Geometry: final body of the model. Coordinates: model frame, mm. A direction names the side the tool comes from. Round coordinates to 2 decimals unless told otherwise and drop trailing zeros. Loops run counter-clockwise (first coordinate to the right, second up) from the corner with the lowest first, then second, coordinate; pieces in that order, holes last. Notation, with made-up numbers: (-2.75, 81.25) -> (33.25, 81.25) arc R8 ccw to (33.25, 86.25) -> close; hole circle Ø6 at (-19, 31). An arc over 180 degrees is marked (long way). Answer in a Markdown table with one row per item.
Autodesk Inventor part; units mm, degrees
ref_plane "Work Plane1" through (1.525, 0, 0) normal (0, 0, 1) x (1, 0, 0)
ref_plane "YZ Plane" through (0, 0, 0) normal (1, 0, 0) x (0, 1, 0)
ref_plane "XZ Plane" through (0, 0, 0) normal (0, 1, 0) x (-1, 0, 0)
sketch "Sketch1" plane through (0, 0, 0) normal (0, 0, 1) x (1, 0, 0)
  line L0 (0, 5.815) -> (0, 4)
  line L1 (38, 4) -> (60, 4)
  line L2 (60, 4) -> (60, 0)
  line L3 (60, 0) -> (-0.6001, 0)
  line L4 (-12.7201, 0) -> (72.12, 0)
  line L5 (-0.6001, 0) -> (-0.6001, 5.815)
  line L6 (-0.6001, 5.815) -> (0, 5.815)
  line L7 (38, 4) -> (37.2331, 4)
  line L8 (37.2331, 4) -> (0, 4)
  line L9 (0, -1.163) -> (0, 6.978)
  dimension "d0" = 60
  dimension "d1" = 22
  dimension "d2" = 8
  dimension "d9" = 0.6001
  dimension "d10" = 11.63
  dimension "d13" = 0.7669
  dimension "d14" = 8
revolve "Body" add sketch "Sketch1" angle 360 about axis through (60, 0, 0) along (-1, 0, 0)
sketch "Sketch2" plane through (-0.6001, 0, 0) normal (-1, 0, 0) x (0, 0, 1)
  line L0 (0, 7.5056) -> (6.5, 3.7528)
  line L1 (6.5, 3.7528) -> (6.5, -3.7528)
  line L2 (6.5, -3.7528) -> (0, -7.5056)
  line L3 (0, -7.5056) -> (-6.5, -3.7528)
  line L4 (-6.5, -3.7528) -> (-6.5, 3.7528)
  line L5 (-6.5, 3.7528) -> (0, 7.5056)
  point P0 (0, 0)
  point P1 (0, 0)
  dimension "d11" = 13
extrude "Head" add sketch "Sketch2" along normal blind 4.7
sketch "Sketch4" plane through (0, 0, 0) normal (0, 0, 1) x (1, 0, 0)
  line L0 (-5.3001, 6.5) -> (-5.3001, 7.5056)
  line L1 (-5.3001, 7.5056) -> (-4.7195, 7.5056)
  line L2 (-4.7195, 7.5056) -> (-5.3001, 6.5)
  line L3 (-6.2401, 0) -> (0.3399, 0)
  line L4 (-0.6001, 7.5056) -> (-5.3001, 7.5056)
  line L5 (-5.3001, 3.7528) -> (-5.3001, 7.5056)
  dimension "d5" = 30
  dimension "d19" = 13
revolve "Chamfer1" cut sketch "Sketch4" angle 360 about axis through (-10, 0, 0) along (1, 0, 0)
thread "Thread"
chamfer "Chamfer2" distance 0.7668 distance2 0.7669 1 edges at (60, -4, 0) measured on face at (60, -0.1514, -1.2467)
ref_plane "Work Plane1" through (1.525, 0, 0) normal (0, 0, 1) x (1, 0, 0)
equation "\"d0\" = NLG"
equation "\"d1\" = GEL"
equation "\"d2\" = GD"
equation "\"d10\" = SD2"
equation "\"d14\" = BDM"
equation "\"d11\" = SW"
equation "\"d3\" = KOH - SD"
equation "\"d5\" = ANG1"
equation "\"d19\" = SW0"
equation "\"d15\" = GEL"
equation "\"d6\" = -0.5 * SPD + 0.5 * GD"
equation "\"NLG\" = 60"
equation "\"GD\" = NND"
equation "\"BDM\" = NND"
equation "\"KOH\" = 5.3"
equation "\"GEL\" = 22"
equation "\"SW\" = 13"
equation "\"SW0\" = SW"
equation "\"SPD\" = NND - 1.2269 * PTC"
equation "\"SD2\" = 11.63"
equation "\"SD\" = 0.6"
equation "\"ANG1\" = 30deg"
equation "\"GAL\" = 0.61345 * PTC"
equation "\"GUL\" = 0.61345 * PTC"
equation "\"RR\" = 0.4"
equation "\"GD1\" = THREADDIA - 1.2269 * PTC"
equation "\"THREADDIA\" = 8"
equation "\"SDH\" = SD2"
equation "\"TOA\" = 30deg"
equation "\"PTC\" = 1.25"
equation "\"NND\" = 8"
equation "\"E0\" = 1.155 * SW"
properties part number "ISO 4014 - M8 x 60" material "Stainless Steel, 440C"
Item 1: Set-up query: faces 4 (the flat face through (-3, 0, -6.5)), 5 (the cylindrical face through (30.031, -0.867, -3.905)). Return all of +Z, -Z, +X, -X, +Y, -Y with unobstructed straight access to the full face (end or side cutting, diameter ignored); none if empty.
Ans:
| item | result |
|---|---|
| face 4 | -Z, +X, -X, +Y, -Y |
| face 5 | +X |
Item 2: Mould query, pull axis Y, two halves, no side actions, for faces 1 (the flat face through (-2.9, 5.6, -3.3)), 2 (the cylindrical face through (-0.296, -1.261, -5.677)), 3 (the flat face through (-5.3, 0, 0)). Classes: released by +Y, released by -Y, zero draft, split by the parting line, or undercut.
Ans:
| item | result |
|---|---|
| face 1 | released by +Y |
| face 2 | split by the parting line |
| face 3 | zero draft |
Item 3: Ray query, L1, parallel to X at y = -3.5, z = -4; L2, parallel to X at y = 6.25, z = -1; L3, parallel to Z at x = -0.5, y = -3. Return the intervals inside material, ascending.
Ans:
| item | result |
|---|---|
| L1 | -5.3 to 0 |
| L2 | -5.3 to -0.6 |
| L3 | -4.98 to 4.98 |
Item 4: Section query A-A, the plane x = 32.5. Output: boundary loops of the cut face in (y, z), and give its area (3 significant figures).
Ans:
| item | result |
|---|---|
| outline | circle Ø8 at (0, 0) |
| area | 50.3 mm2 |
Item 5: First-contact query: P1, Ø4, axis at x = 17, z = -1, coming from the -Y side; P2, Ø8, axis at x = 8, y = 4.5, coming from the -Z side; P3, Ø5, axis at x = 47, z = -4, coming from the +Y side. Flat tips, straight axial feed; report the tip coordinate or a pass-through.
Ans:
| item | result |
|---|---|
| P1 | y = -4 |
| P2 | z = -3.97 |
| P3 | y = 3.71 |
